```python
from build123d import *

# Parameters (mm, degrees)
F0_W      = 88
F0_H      = 88
F1_DEPTH  = 1700
F3_DEPTH  = 88.001
F5_DEPTH  = 88.001
F7_DEPTH  = 31
F9_DEPTH  = 31
F11_DEPTH = 31
F13_DEPTH = 25.0000003725
F14_R     = 5


with BuildPart() as f1:
    # F0 (on Top) → F1 (new body)
    with BuildSketch(Plane.XY):
        with Locations((44, 44)):
            Rectangle(F0_W, F0_H)
    extrude(amount=F1_DEPTH)

    # F2 (on face) → F3 (cut, through all)
    with BuildSketch(Plane(origin=(0, 0, 0), x_dir=(0, -1, 0), z_dir=(-1, 0, 0))):
        Polygon((-88, 1663.5492065112), (0, 1700), (-88, 1700), align=None)
    extrude(amount=-F3_DEPTH, mode=Mode.SUBTRACT)

    # F4 (on face) → F5 (cut, through all)
    with BuildSketch(Plane(origin=(0, 0, 0), x_dir=(0, -1, 0), z_dir=(-1, 0, 0))):
        Polygon((-65, 1594.0761184457), (-65, 1673.0761184457), (-88, 1663.5492065112), (-88, 1584.5492065112), align=None)
    extrude(amount=-F5_DEPTH, mode=Mode.SUBTRACT)

    # F6 (on face) → F7 (cut)
    with BuildSketch(Plane.YZ.offset(88)):
        Polygon((29, 282), (44, 282), (59, 282), (59, 370), (29, 370), align=None)
    extrude(amount=-F7_DEPTH, mode=Mode.SUBTRACT)

    # F8 (on face) → F9 (cut)
    with BuildSketch(Plane.YZ.offset(88)):
        Polygon((29, 1460), (44, 1460), (59, 1460), (59, 1548), (29, 1548), align=None)
    extrude(amount=-F9_DEPTH, mode=Mode.SUBTRACT)

    # F10 (on face) → F11 (cut)
    with BuildSketch(Plane.XZ):
        Polygon((29, 162), (44, 162), (59, 162), (59, 250), (29, 250), align=None)
    extrude(amount=-F11_DEPTH, mode=Mode.SUBTRACT)

    # F12 (on face) → F13 (cut)
    with BuildSketch(Plane.XZ):
        Polygon((29, 1056), (44, 1056), (59, 1056), (59, 1144), (29, 1144), align=None)
    extrude(amount=-F13_DEPTH, mode=Mode.SUBTRACT)

    # F14
    f14_edges = [f1.edges().sort_by_distance(p)[0] for p in [
        (88, 0, 850),
        (0, 0, 850),
        (88, 88, 792.274603),
        (0, 88, 792.274603),
    ]]
    fillet(f14_edges, radius=F14_R)


solid = f1.part
```
Read the model definition and answer for the solid it produces. Units are mm, in the model's axes. A direction names the side the tool comes from. Coordinates: 2 decimals unless noted, no trailing zeros. Loops run counter-clockwise (first coordinate to the right, second up) from the corner with the lowest first, then second, coordinate; pieces in that order, holes last. Notation, with made-up numbers: (54, 22) -> (102, 22) arc R13 ccw to (102, 32) -> close; hole circle Ø7 at (57.25, 87). An arc over 180 degrees is marked (long way). Return JSON: item names as keys, results as strings.
Item 1: For a pull along Z with two mould halves and no side action, classify faces 5 (the flat face through (44, 31, 207)), 6 (the flat face through (43.384, 32.955, 1686.35)), 7 (the flat face through (43, 0, 838)) as +Z half, -Z half, draft (parallel to the pull), parting line (faces both ways), or undercut.
Answers:
{"face 5": "undercut", "face 6": "+Z half", "face 7": "draft"}
Item 2: Find section A-A (z = 1519). Determine the outline of the cut face in (x, y).
Answers:
{"outline": "(0, 5) arc R5 ccw to (5, 0) -> (83, 0) arc R5 ccw to (88, 5) -> (88, 29) -> (57, 29) -> (57, 59) -> (88, 59) -> (88, 83) arc R5 ccw to (83, 88) -> (5, 88) arc R5 ccw to (0, 83) -> close"}
Item 3: For faces 1 (the flat face through (73, 59, 325)), 2 (the flat face through (44, 25, 1101)), 3 (the flat face through (0, 43, 837)), 4 (the flat face through (43, 65, 1633)), determine the directions among +Z, -Z, +X, -X, +Y, -Y from which every point of the face is accessible in a straight line to the end or side of a thin tool.
Answers:
{"face 1": "+X", "face 2": "-Y", "face 3": "+Z, -Z, -X, +Y, -Y", "face 4": "+Z, +X, -X, +Y"}
Item 4: Flat-ended cylindrical pins translate along their axes: P1, Ø20, axis at x = 37, y = 13.5, coming from the +Z side; P2, Ø15, axis at x = 77.5, y = 49, coming from the -Z side; P3, Ø9, axis at x = 50.5, y = 23, coming from the +Z side; P4, Ø1.5, axis at x = 53, z = 1067.5, coming from the -Y side. Find the tip coordinate at first contact, or state that the pin passes through.
Answers:
{"P1": "stops at z = 1698.55", "P2": "stops at z = 0", "P3": "stops at z = 1692.34", "P4": "stops at y = 25"}
Item 5: Find the intervals of material crossed by probe 1 along Z at (x, y) = (33.5, 22.5); probe 2 along Z at (x, y) = (32.5, 11.5); probe 3 along Y at (x, z) = (74, 1611), in increasing order.
Answers:
{"probe 1": "z = 0 to 162, 250 to 1056, 1144 to 1690.68", "probe 2": "z = 0 to 162, 250 to 1056, 1144 to 1695.24", "probe 3": "y = 0 to 65"}
